Answer from the drawing. Dimensions are ordinates in mm from the lowest x, y and z of the part. A direction names the side the tool comes from. Round coordinates to 2 decimals unless told otherwise and drop trailing zeros. Order: outer loops, then holes, each group sorted by start corner. A loop starts at its lowest first (then second) coordinate and runs counter-clockwise, first axis right, second up. Notation, with made-up numbers: (38, -31.5) -> (80, -31.5) arc R13 cw to (80, -18.5) -> close; hole circle Ø10 at (67, 70). An arc over 180 degrees is marked (long way). Use a Markdown table: item, result. Add a question column.
Item 1: For a pull along Y with two mould halves and no side action, classify the marked faces 1, 2 and 3 as +Y half, -Y half, draft (parallel to the pull), parting line (faces both ways), or undercut.
Item 2: A cutting plane is placed at B-B, the plane x = 6.35. Determine the outline of the cut face in (y, z), plus the area to 3 significant figures.
Item 3: Flat-ended cylindrical pins translate along their axes: P1, Ø6, axis at y = 5, z = 8.5, coming from the -X side; P2, Ø1, axis at x = 5.5, z = 6.5, coming from the +Y side. Find the tip coordinate at first contact, or state that the pin passes through.
Item 4: A cutting plane is placed at D-D, the plane x = 11. Determine the outline of the cut face in (y, z), plus the area to 3 significant figures.
Item 5: A tool of negligible diameter and unlimited length cuts with its end or side. For the marked faces 4 and 5, from which of +Z, -Z, +X, -X, +Y, -Y can it reach the whole face along a straight path? Write none if from no direction.
Item 6: A cutting plane is placed at A-A, the plane y = 16.5. Give the number of separate pieces and of enclosed holes in the cut face, plus the area to 3 significant figures.
Item 7: A cutting plane is placed at C-C, the plane z = 9. Determine the outline of the cut face in (x, y) (3 decimals).
Item 8: Find the intervals of material crossed by L1, parallel to X at y = 11.75, z = 5.25; L2, parallel to X at y = 12.25, z = 6.35; L3, parallel to X at y = 9.25, z = 8.75, in increasing order. Write a range as [from, to].
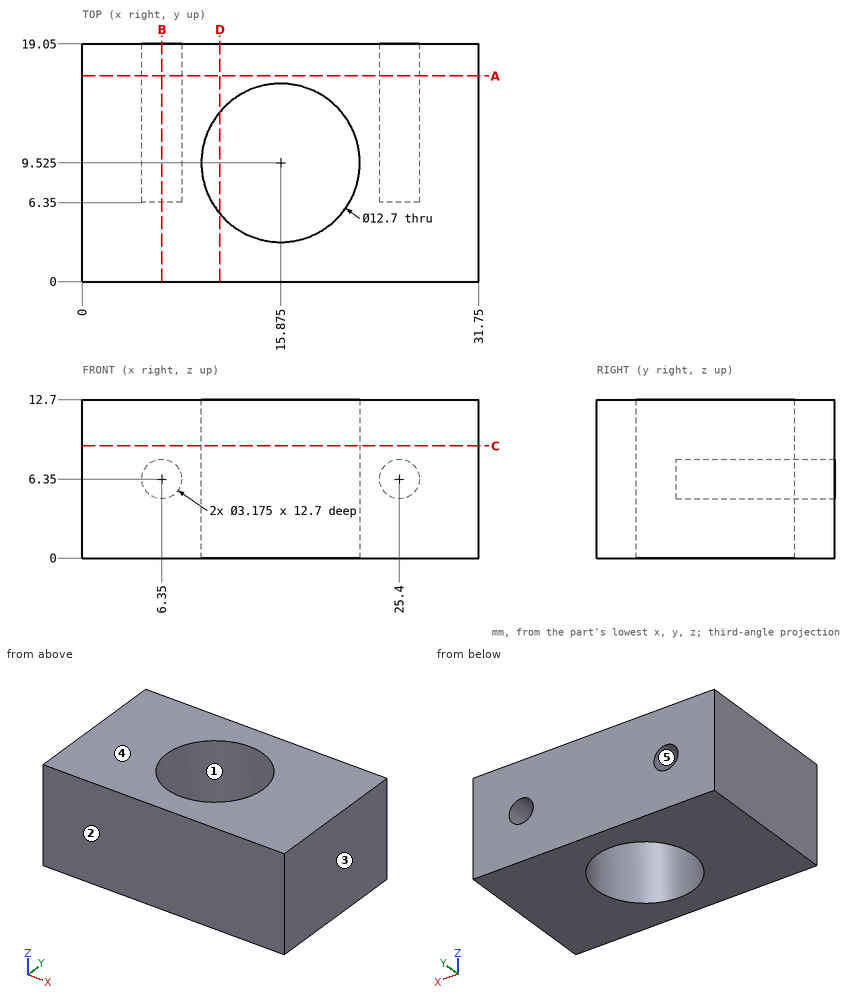
Reported:
| question | item | result |
|---|---|---|
| 1 | face 1 | undercut |
| 1 | face 2 | -Y half |
| 1 | face 3 | draft |
| 2 | outline | (0, 0) -> (19.05, 0) -> (19.05, 4.76) -> (6.35, 4.76) -> (6.35, 7.94) -> (19.05, 7.94) -> (19.05, 12.7) -> (0, 12.7) -> close |
| 2 | area | 202 mm² |
| 3 | P1 | x = 0 |
| 3 | P2 | y = 6.35 |
| 4 | outline | (0, 0) -> (5.46, 0) -> (5.46, 12.7) -> (0, 12.7) -> close; (13.59, 0) -> (19.05, 0) -> (19.05, 12.7) -> (13.59, 12.7) -> close |
| 4 | area | 139 mm² |
| 5 | face 4 | +Z, +X, -X, +Y, -Y |
| 5 | face 5 | +Y |
| 6 | separate pieces | 1 |
| 6 | enclosed holes | 2 |
| 6 | area | 387 mm² |
| 7 | outline | (0, 0) -> (31.75, 0) -> (31.75, 19.05) -> (0, 19.05) -> close; hole circle Ø12.7 at (15.875, 9.525) |
| 8 | L1 | [0, 5.21], [7.49, 9.93], [21.82, 24.26], [26.54, 31.75] |
| 8 | L2 | [0, 4.76], [7.94, 10.14], [21.61, 23.81], [26.99, 31.75] |
| 8 | L3 | [0, 9.53], [22.22, 31.75] |
